Geometry: final body of the model. Coordinates: model frame, mm. Face numbers are marked on the shaded views. A direction names the side the tool comes from. Coordinates: 2 decimals unless noted, no trailing zeros. Loops run counter-clockwise (first coordinate to the right, second up) from the corner with the lowest first, then second, coordinate; pieces in that order, holes last. Notation, with made-up numbers: (-22, 46) - (2, 46) arc R21 cw to (2, 50) - close; hole circle Ø7 at (73, -21). An arc over 180 degrees is marked (long way). Put each result on its own line as item: value. Start each with the question number.
1) Reachability of the marked faces 1, 2 and 3 from +Z, -Z, +X, -X, +Y, -Y: full face, straight path, thin tool, end or side. Return the list, or none.
2) Section D-D on y = 41.91. Output: boundary loops of the cut face in (x, z), and give its area (3 significant figures).
3) Material intervals for line 1 along Y through (x, z) = (3.75, 2.95) (3 decimals); line 2 along Y through (x, z) = (-1.5, 1.4); line 3 along Y through (x, z) = (2.25, 3.5), sorted ascending. Write a range as from..to.
4) Contact query for flat-ended pins moving along their axis: pin 1 Ø1.9 at (x, z) = (3, 1.5) entering from +Y; pin 2 Ø1.6 at (x, z) = (4, 1.5) entering from -Y; pin 3 Ø1.5 at (x, z) = (6.5, 3) entering from +Y. Output: stop coordinate, or through.
5) Section C-C on y = 35.5. Output: boundary loops of the cut face in (x, z), and give its area (3 significant figures).
6) Draft query along Y for the marked faces 4 and 5. Return one class per face: +Y half, -Y half, draft (parallel to the pull), parting line (faces both ways), or undercut.
7) Section B-B on x = -1.25. Output: boundary loops of the cut face in (y, z).
Autodesk Inventor part; units mm, degrees
ref_plane "YZ Plane" through (0, 0, 0) normal (1, 0, 0) x (0, 1, 0)
ref_plane "XZ Plane" through (0, 0, 0) normal (0, 1, 0) x (-1, 0, 0)
ref_plane "XY Plane" through (0, 0, 0) normal (0, 0, 1) x (1, 0, 0)
sketch "Sketch1" plane through (0, 0, 0) normal (0, 0, 1) x (1, 0, 0)
  arc A0 (0, -1.7145) -> (0, 1.7145) centre (0, 0) ccw
  arc A1 (-3.0427, -1.7145) -> (0, 3.4925) centre (0, 0) ccw
  arc A2 (0, 40.1955) -> (0, 43.6245) centre (0, 41.91) ccw
  arc A3 (0, 38.4175) -> (-3.0427, 43.6245) centre (0, 41.91) ccw
  line L0 (0, 40.1955) -> (-3.0427, 40.1955)
  line L1 (-3.0427, 1.7145) -> (0, 1.7145)
  line L2 (-3.0427, 29.337) -> (6.4823, 29.337)
  line L3 (6.4823, 29.337) -> (6.4823, 12.573)
  line L4 (6.4823, 12.573) -> (-3.0427, 12.573)
  line L5 (0, 3.4925) -> (0, 10.795)
  line L6 (0, 10.795) -> (8.3873, 10.795)
  line L7 (8.3873, 10.795) -> (8.3873, 31.115)
  line L8 (8.3873, 31.115) -> (0, 31.115)
  line L9 (0, 31.115) -> (0, 38.4175)
  line L10 (0, 43.6245) -> (-3.0427, 43.6245)
  line L11 (0, -1.7145) -> (-3.0427, -1.7145)
  line L12 (-3.0427, 40.1955) -> (-3.0427, 29.337)
  line L13 (-3.0427, 12.573) -> (-3.0427, 1.7145)
  point P0 (8.3873, 20.955)
  point P1 (6.4823, 20.955)
  dimension "d0" = 3.429
  dimension "d1" = 6.985
  dimension "d2" = 41.91
  dimension "d5" = 20.955
  dimension "d6" = 16.764
  dimension "d7" = 9.525
  dimension "d8" = 20.32
  dimension "d9" = 11.43
extrude "Extrusion1" add sketch "Sketch1" along normal blind 3.81
fillet "Fillet1" radius 3.175 8 edges at (0, 31.115, 1.905) (8.3873, 31.115, 1.905) (8.3873, 10.795, 1.905) (0, 10.795, 1.905) (-3.0427, 12.573, 1.905) (-3.0427, 29.337, 1.905) (0, 3.4925, 1.905) (0, 38.4175, 1.905)
fillet "Fillet2" radius 0.508 4 edges at (-3.0427, -1.7145, 1.905) (-3.0427, 1.7145, 1.905) (-3.0427, 40.1955, 1.905) (-3.0427, 43.6245, 1.905)
properties part number "batteryConnectorHolder" material "ABS Plastic"
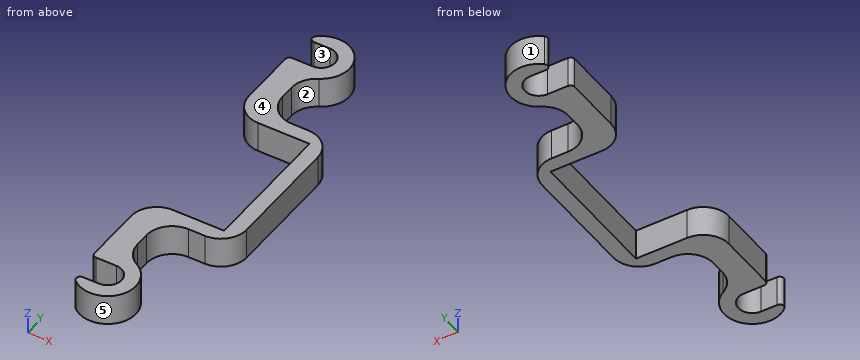
Answer block:
1. face 1: +Z, -Z
1. face 2: +Z, -Z, +X
1. face 3: +Z, -Z, -X
2. outline: (1.71, 0) - (3.49, 0) - (3.49, 3.81) - (1.71, 3.81) - close
2. area: 6.77 mm²
3. line 1: y = 10.795..12.573, 29.337..31.115
3. line 2: y = -3.15..-1.71, 1.71..12.12, 29.79..40.2, 43.62..45.06
3. line 3: y = -2.67..2.67, 10.66..12.57, 29.34..31.25, 39.24..44.58
4. pin 1: stops at y = 44.74
4. pin 2: stops at y = -1.4
4. pin 3: stops at y = 31.07
5. outline: (-3.04, 0) - (0, 0) - (0, 3.81) - (-3.04, 3.81) - close
5. area: 11.6 mm²
6. face 4: draft
6. face 5: undercut
7. outline: (-3.26, 0) - (-1.71, 0) - (-1.71, 3.81) - (-3.26, 3.81) - close; (1.71, 0) - (12.26, 0) - (12.26, 3.81) - (1.71, 3.81) - close; (29.65, 0) - (40.2, 0) - (40.2, 3.81) - (29.65, 3.81) - close; (43.62, 0) - (45.17, 0) - (45.17, 3.81) - (43.62, 3.81) - close
